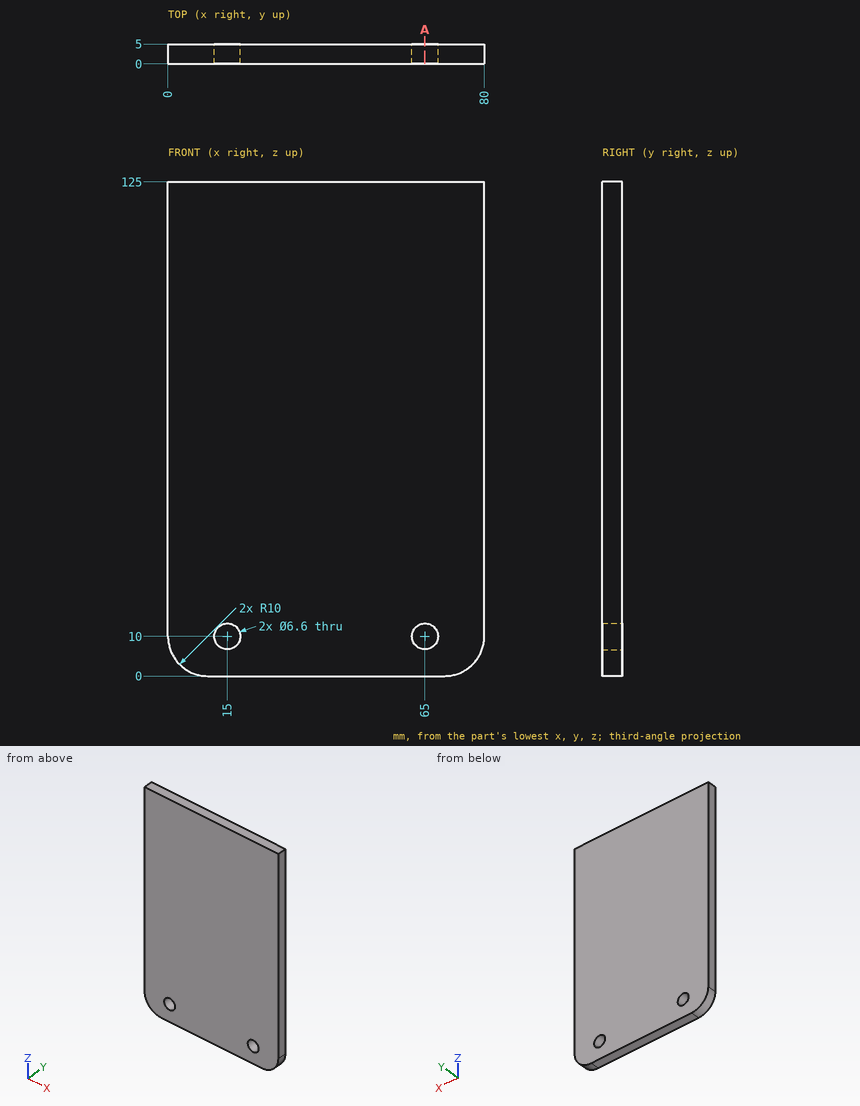
Input: dimensioned drawing with shaded views. Units: mm. Origin: part minimum x, y, z. Coordinates: 2 decimals unless noted, no trailing zeros. Order: outer loops, then holes, each group sorted by start corner. A loop starts at its lowest first (then second) coordinate and runs counter-clockwise, first axis right, second up. Notation, with made-up numbers: (38.25, 22.5) - (71.25, 22.5) arc R18 ccw to (71.25, 51.5) - close; hole circle Ø10 at (77.25, 63.25). An arc over 180 degrees is marked (long way). Return JSON: item names as keys, results as strings. Group by question number.
1. Cut plane A-A (x = 65). Output: boundary loops of the cut face in (y, z), plus the area to 3 significant figures.
2. Pin query (flat end, axial travel): pin 1 (6 mm diameter, centred on x = 65, z = 10, fed in from +Y). Return the tip coordinate at first contact, or that it passes through.
3. Material intervals for line 1 along Z through (x, y) = (65, 1.5); line 2 along X through (y, z) = (2.85, 11); line 3 along Z through (x, y) = (62, 2.1), sorted ascending. Write a range as [from, to].
Resolved:
{
 "1": {"outline": "(0, 0) - (5, 0) - (5, 6.7) - (0, 6.7) - close; (0, 13.3) - (5, 13.3) - (5, 125) - (0, 125) - close", "area": "592 mm²"},
 "2": {"pin 1": "passes through"},
 "3": {"line 1": "z = [0, 6.7], [13.3, 125]", "line 2": "x = [0, 11.86], [18.14, 61.86], [68.14, 80]", "line 3": "z = [0, 8.63], [11.37, 125]"}
}
